```python
from build123d import *

# Parameters (mm, degrees)
SKETCH1_R           = 1.2192
SKETCH1_R_2         = 3.8735
BOSS_EXTRUDE1_DEPTH = 3


with BuildPart() as part:
    # Sketch1 → Boss-Extrude1 (new body)
    with BuildSketch(Plane(origin=(22.066943297, 0, -12.337708943), x_dir=(0, -1, 0), z_dir=(-0.872839337, 0, 0.488007675))):
        with BuildLine():
            ThreePointArc((-72.947857894, 167.897835008), (-47.979019161, 146.065099757), (-37.424383054, 114.621326243))
            ThreePointArc((-37.424383054, 114.621326243), (-20.859592098, 104.154397101), (-16.22026224, 123.191873917))
            ThreePointArc((-16.22026224, 123.191873917), (-38.39182686, 152.45760543), (-56.883606586, 184.176927637))
            ThreePointArc((-56.883606586, 184.176927637), (-76.241477877, 187.213656824), (-72.947857894, 167.897835008))
        make_face()
        with Locations((-32.452983518, 110.624678087)):
            Circle(SKETCH1_R, mode=Mode.SUBTRACT)
        with Locations((-20.665274094, 108.268060476)):
            Circle(SKETCH1_R, mode=Mode.SUBTRACT)
        with Locations((-18.308656482, 120.055769899)):
            Circle(SKETCH1_R, mode=Mode.SUBTRACT)
        with Locations((-30.096365906, 122.412387511)):
            Circle(SKETCH1_R, mode=Mode.SUBTRACT)
        with Locations((-62.938209154, 171.667105905)):
            Circle(SKETCH1_R, mode=Mode.SUBTRACT)
        with Locations((-60.581591542, 183.454815329)):
            Circle(SKETCH1_R, mode=Mode.SUBTRACT)
        with Locations((-72.369300966, 185.811432941)):
            Circle(SKETCH1_R, mode=Mode.SUBTRACT)
        with Locations((-74.725918578, 174.023723517)):
            Circle(SKETCH1_R, mode=Mode.SUBTRACT)
        with Locations((-67.65375506, 178.739269423)):
            Circle(SKETCH1_R_2, mode=Mode.SUBTRACT)
        with Locations((-25.38082, 115.340223993)):
            Circle(SKETCH1_R_2, mode=Mode.SUBTRACT)
    extrude(amount=-BOSS_EXTRUDE1_DEPTH)


solid = part.part
```
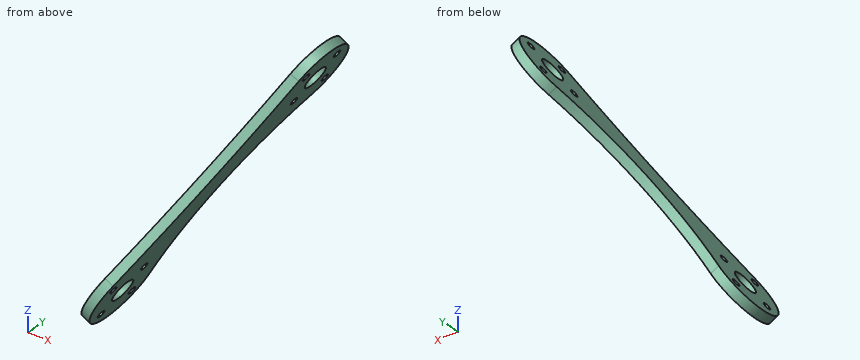
Source: CAD feature listing. Evaluate the final solid. Frame: model axes, mm. Give positions to 0.01 mm unless a question says otherwise; leave off trailing zeros. Write each loop counter-clockwise with the first axis right and the second up, starting at its lowest first coordinate (ties: lowest second). Pieces come first, ordered by that corner, then holes.
1. Section query B-B (y = 74.5). Return the cut outline in (x, z) (3 decimals), then the cut area to 3 significant figures.
2. Section query A-A (y = 23). Return the cut outline in (x, z).
3. First-contact query: pin 1 (5 mm diameter, centred on y = 55.5, z = 127.5, fed in from -X); pin 2 (10 mm diameter, centred on x = 99, y = 39.5, fed in from -Z); pin 3 (10 mm diameter, centred on y = 30.5, z = 122, fed in from +X); pin 4 (10 mm diameter, centred on x = 78.5, y = 26, fed in from +Z). Flat tips, straight axial feed; report the tip coordinate or a pass-through.
4. Material intervals for line 1 along Z through (x, y) = (82.5, 36.5); line 2 along Y through (x, z) = (99, 122); line 3 along X through (y, z) = (35, 103), sorted ascending.
Output values:
1. outline: (104.445, 135.002) - (107.064, 133.538) - (109.026, 137.047) - (106.407, 138.511) - close; (107.577, 140.603) - (110.195, 139.139) - (116.76, 150.88) - (114.141, 152.344) - close
1. area: 52.4 mm2
2. outline: (72.58, 78.01) - (75.2, 76.55) - (79.48, 84.2) - (76.86, 85.67) - close; (79.84, 91) - (82.46, 89.54) - (88.8, 100.88) - (86.18, 102.34) - close
3. pin 1: stops at x = 98.85
3. pin 2: stops at z = 110.17
3. pin 3: passes through
3. pin 4: stops at z = 97.54
4. line 1: z = 89.6 to 95.75
4. line 2: y = 39.94 to 54.99
4. line 3: x = 86.55 to 89.99
